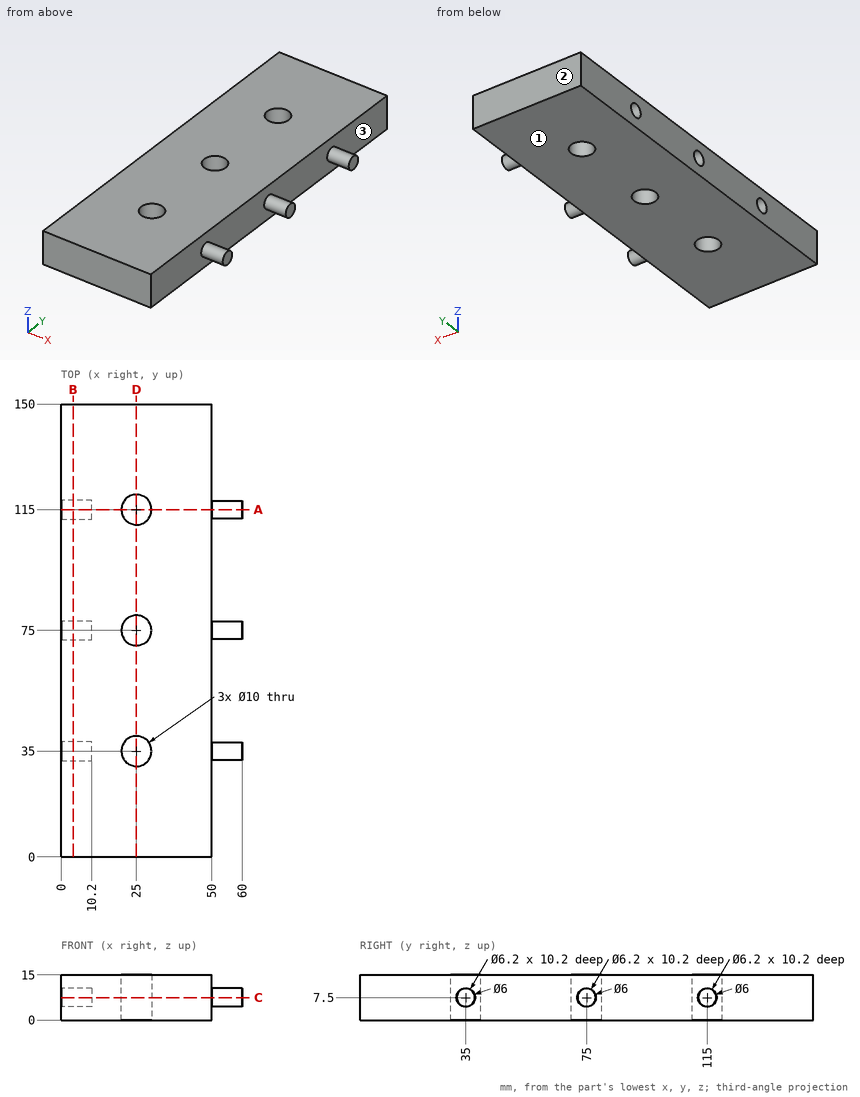
Study the drawing (mm; zero at the part's minimum x, y, z) and answer. Coordinates: 2 decimals unless noted, no trailing zeros. Loops run counter-clockwise (first coordinate to the right, second up) from the corner with the lowest first, then second, coordinate; pieces in that order, holes last. Notation, with made-up numbers: (-2.5, -6.5) -> (55.5, -6.5) arc R21 ccw to (55.5, 8.5) -> close; hole circle Ø9 at (15.5, -20). An arc over 180 degrees is marked (long way). Write each question's results on one line, items separated by ' | '. Start each with the question number.
1) Find section A-A on y = 115. Determine the outline of the cut face in (x, z), then the cut area to 3 significant figures.
2) Consider line 1 along Y through (x, z) = (25, 6.5); line 2 along Y through (x, z) = (21.5, 7.25); line 3 along X through (y, z) = (48.5, 8.25). Determine where each line is inside the solid, lowest interval first.
3) Find section C-C on z = 7.5. Count the separate pieces of the cut face and the enclosed holes in it, then the cut area to 3 significant figures.
4) The mould has two halves that part along Y. Classify the marked faces 1, 2 and 3: pulls with the +Y half, pulls with the -Y half, needs draft (parallel to the pull), parting line crosses it, or undercut.
5) Find section D-D on x = 25. Determine the outline of the cut face in (y, z), then the cut area to 3 significant figures.
6) Flat-ended cylindrical pins translate along their axes: P1, Ø1.9, axis at y = 36, z = 8, coming from the -X side; P2, Ø1, axis at x = 51.5, z = 2, coming from the +Y side; P3, Ø4.5, axis at y = 89, z = 7.5, coming from the +X side. Find the tip coordinate at first contact, or state that the pin passes through.
7) Find section B-B on x = 4. Determine the outline of the cut face in (y, z), then the cut area to 3 significant figures.
Response values:
1) outline: (0, 0) -> (20, 0) -> (20, 15) -> (0, 15) -> (0, 10.6) -> (10.2, 10.6) -> (10.2, 4.4) -> (0, 4.4) -> close; (30, 0) -> (50, 0) -> (50, 4.5) -> (60, 4.5) -> (60, 10.5) -> (50, 10.5) -> (50, 15) -> (30, 15) -> close | area: 597 mm^2
2) line 1: y = 0 to 30, 40 to 70, 80 to 110, 120 to 150 | line 2: y = 0 to 31.43, 38.57 to 71.43, 78.57 to 111.43, 118.57 to 150 | line 3: x = 0 to 50
3) separate pieces: 1 | enclosed holes: 3 | area: 7,250 mm^2
4) face 1: needs draft | face 2: pulls with the +Y half | face 3: undercut
5) outline: (0, 0) -> (30, 0) -> (30, 15) -> (0, 15) -> close; (40, 0) -> (70, 0) -> (70, 15) -> (40, 15) -> close; (80, 0) -> (110, 0) -> (110, 15) -> (80, 15) -> close; (120, 0) -> (150, 0) -> (150, 15) -> (120, 15) -> close | area: 1,800 mm^2
6) P1: stops at x = 10.2 | P2: passes through | P3: stops at x = 50
7) outline: (0, 0) -> (150, 0) -> (150, 15) -> (0, 15) -> close; hole circle Ø6.2 at (35, 7.5); hole circle Ø6.2 at (75, 7.5); hole circle Ø6.2 at (115, 7.5) | area: 2,160 mm^2
